Here's how the part is built. I have some questions about the finished solid (model axes, mm). A direction names the side the tool comes from. Coordinates: 2 decimals unless noted, no trailing zeros. Order: outer loops, then holes, each group sorted by start corner. A loop starts at its lowest first (then second) coordinate and runs counter-clockwise, first axis right, second up. Notation, with made-up numbers: (-18.5, 64) - (34.5, 64) arc R19 cw to (34.5, 68) - close; hole circle Ø3 at (63.25, 60.25). An arc over 180 degrees is marked (long way). Answer as CSV lines item,"result". Start each with the question number.
Item 1: I'm going to push flat-ended pins straight in: pin 1 (0.6 mm diameter, centred on x = -4, z = 0.5, fed in from +Y); pin 2 (5 mm diameter, centred on x = -3.5, z = 2.5, fed in from -Y); pin 3 (1.5 mm diameter, centred on y = 3.5, z = -0.5, fed in from +X). Where does each tip first touch, or does it pass through?
Item 2: Imagine slicing it at B-B on z = 0. List the corners of the cut face in (x, y) for me, and give its area (3 significant figures).
Item 3: On a 3-axis mill with a long thin cutter (end or side, diameter ignored), from which of +Z, -Z, +X, -X, +Y, -Y can I reach the whole of each face in a straight line? I mean faces 3 (the face through (-4, 0.84, -2)), 4 (the face through (2.984, 2.575, 3.174)). Say none if no direction works.
Item 4: We'd pull the mould along Z, two halves only. Please class faces 1 (the face through (-4, -0.04, -2)), 2 (the face through (-0.35, 2.57, -2.86)): pulls with the +Z half, pulls with the -Z half, needs draft (parallel to the pull), parting line crosses it, or undercut.
Item 5: I need wall thicknesses on line 1 (Y direction, x = 4.5, z = 3); line 2 (Y direction, x = -1.75, z = 3); line 3 (X direction, y = 0.7, z = -0.66). Which ranges of each line are inside material? Lowest first, please.
Item 6: Imagine slicing it at A-A on y = 1.6. List the corners of the cut face in (x, z) for me, and give its area (3 significant figures).
from build123d import *

# Parameters (mm, degrees)
SKETCH_1_W               = 9.5
SKETCH_1_H               = 9
EXTRUDE_1_DEPTH          = 0.8
SKETCH_4_R               = 0.4
CUT_EXTRUDE_1_DEPTH      = 7.59185103
EXTRUDE_2_DEPTH          = 0.04
EXTRUDE_2_DEPTH_BACK     = 0.84
SKETCH_6_W               = 1.3
SKETCH_6_H               = 0.8
SKETCH_6_W_2             = 0.8
SKETCH_6_H_2             = 1
CUT_EXTRUDE_2_DEPTH      = 7.62568487
CUT_EXTRUDE_2_DEPTH_BACK = 7.62568487
SKETCH_5_R               = 0.4
SKETCH_5_R_2             = 0.3
SKETCH_7_R               = 4
SKETCH_7_R_2             = 3
EXTRUDE_3_DEPTH          = 3.8
CHAMFER_1_SIZE           = 0.2
CHAMFER_2_SIZE           = 0.2


with BuildPart() as part:
    # Эскиз1 → Бобышка-Вытянуть1 (new body)
    with BuildSketch(Plane(origin=(0, 0, 0), x_dir=(1, 0, 0), z_dir=(0, 1, 0))):
        Rectangle(SKETCH_1_W, SKETCH_1_H)
    extrude(amount=EXTRUDE_1_DEPTH)

    # Эскиз4 → Вырез-Вытянуть1 (cut, through all)
    with BuildSketch(Plane.XZ):
        with Locations((-4.75, -4.5)):
            Circle(SKETCH_4_R)
        with Locations((4.75, -4.5)):
            Circle(SKETCH_4_R)
        with Locations((-4.75, 4.5)):
            Circle(SKETCH_4_R)
        with Locations((4.75, 4.5)):
            Circle(SKETCH_4_R)
    extrude(amount=-CUT_EXTRUDE_1_DEPTH, mode=Mode.SUBTRACT)

    # Эскиз6 → Бобышка-Вытянуть2 (add, two sides: drawn at the far end of the back side and taken through both)
    with BuildSketch(Plane(origin=(0, 0.8, 0), x_dir=(1, 0, 0), z_dir=(0, 1, 0)).offset(-EXTRUDE_2_DEPTH_BACK)):
        with Locations((-4.14, 3.2)):
            Rectangle(SKETCH_6_W, SKETCH_6_H)
        with Locations((-4.14, 1.93)):
            Rectangle(SKETCH_6_W, SKETCH_6_H)
        with Locations((-4.14, 0.66)):
            Rectangle(SKETCH_6_W, SKETCH_6_H)
        with Locations((-4.14, -0.61)):
            Rectangle(SKETCH_6_W, SKETCH_6_H)
        with Locations((-4.14, -1.88)):
            Rectangle(SKETCH_6_W, SKETCH_6_H)
        with Locations((-4.14, -3.15)):
            Rectangle(SKETCH_6_W, SKETCH_6_H)
        with Locations((3.15, 4)):
            Rectangle(SKETCH_6_W_2, SKETCH_6_H_2)
        with Locations((3.15, -4)):
            Rectangle(SKETCH_6_W_2, SKETCH_6_H_2)
    extrude(amount=EXTRUDE_2_DEPTH + EXTRUDE_2_DEPTH_BACK)

    # Эскиз5 → Вырез-Вытянуть2 (cut, two sides: drawn at the far end of the back side and taken through both)
    with BuildSketch(Plane.XZ.offset(-CUT_EXTRUDE_2_DEPTH_BACK)):
        with Locations((3.15, 4.5)):
            Circle(SKETCH_5_R)
        with Locations((3.15, -4.5)):
            Circle(SKETCH_5_R)
        with Locations((-4.75, -3.2)):
            Circle(SKETCH_5_R_2)
        with Locations((-4.75, -1.93)):
            Circle(SKETCH_5_R_2)
        with Locations((-4.75, -0.66)):
            Circle(SKETCH_5_R_2)
        with Locations((-4.75, 0.61)):
            Circle(SKETCH_5_R_2)
        with Locations((-4.75, 1.88)):
            Circle(SKETCH_5_R_2)
        with Locations((-4.75, 3.15)):
            Circle(SKETCH_5_R_2)
    extrude(amount=CUT_EXTRUDE_2_DEPTH + CUT_EXTRUDE_2_DEPTH_BACK, mode=Mode.SUBTRACT)

    # Эскиз7 → Бобышка-Вытянуть3 (add)
    with BuildSketch(Plane(origin=(0, 0.8, 0), x_dir=(1, 0, 0), z_dir=(0, 1, 0))):
        with Locations(Location((0.55, 0, 0), (0, 0, 90))):
            Circle(SKETCH_7_R)
        with Locations(Location((0.55, 0, 0), (0, 0, 90))):
            Circle(SKETCH_7_R_2, mode=Mode.SUBTRACT)
    extrude(amount=EXTRUDE_3_DEPTH)

    # Фаска1
    chamfer_1_edges = [part.edges().sort_by_distance(p)[0] for p in [
        (0.55, 4.6, 4),
    ]]
    chamfer(chamfer_1_edges, length=CHAMFER_1_SIZE)

    # Фаска2
    chamfer_2_edges = [part.edges().sort_by_distance(p)[0] for p in [
        (0.55, 4.6, 3),
    ]]
    chamfer(chamfer_2_edges, length=CHAMFER_2_SIZE)


solid = part.part
Responses:
1,pin 1,"stops at y = 0.84"
1,pin 2,"stops at y = -0.04"
1,pin 3,"stops at x = 4.55"
2,outline,"(-4.75, 0) - (4.75, 0) - (4.75, 0.8) - (4.55, 0.8) - (4.55, 4.4) - (4.35, 4.6) - (3.75, 4.6) - (3.55, 4.4) - (3.55, 0.8) - (-2.45, 0.8) - (-2.45, 4.4) - (-2.65, 4.6) - (-3.25, 4.6) - (-3.45, 4.4) - (-3.45, 0.8) - (-4.75, 0.8) - close"
2,area,"15.1 mm^2"
3,face 3,"+Z, -Z, -X, +Y"
3,face 4,"+Y"
4,face 1,"needs draft"
4,face 2,"undercut"
5,line 1,"y = 0 to 0.8"
5,line 2,"y = 0 to 4.6"
5,line 3,"x = -4.45 to 4.75"
6,outline,"circle Ø8 at (0.55, 0); hole circle Ø6 at (0.55, 0)"
6,area,"22.0 mm^2"
